Read the model definition and answer for the solid it produces. Units are mm, in the model's axes. Face numbers are marked on the shaded views. A direction names the side the tool comes from. Round coordinates to 2 decimals unless told otherwise and drop trailing zeros. Order: outer loops, then holes, each group sorted by start corner. A loop starts at its lowest first (then second) coordinate and runs counter-clockwise, first axis right, second up. Notation, with made-up numbers: (55, -5) - (112, -5) arc R22 ccw to (112, 27) - close; hole circle Ø9 at (86.5, -28). An arc over 180 degrees is marked (long way). Answer as a JSON object with one key per item and string values. Group by question number.
Q1. A cutting plane is placed at C-C on z = 29. Determine the outline of the cut face in (x, y) (3 decimals).
Q2. A cutting plane is placed at B-B on x = 45.5. Determine the outline of the cut face in (y, z), and give its area (3 significant figures).
Q3. Consider line 1 (Z direction, x = 39.5, y = -51); line 2 (Z direction, x = 9.5, y = -12); line 3 (Y direction, x = 93.5, z = 32). Determine where each line is inside the solid, lowest interval first.
Q4. Given pin 1 Ø0.9 at (x, z) = (16.5, 9.5) entering from +Y; pin 2 Ø0.6 at (x, z) = (20.5, 8.5) entering from +Y; pin 3 Ø5 at (x, z) = (18.5, 19.5) entering from +Y; pin 4 Ø4.5 at (x, z) = (108, 20.5) entering from -Y, each flat-ended and moving along its own axis, determine where each tip first touches the part or whether it passes through.
Q5. The mould has two halves that part along Z. Classify the marked faces 1, 2 and 3: pulls with the +Z half, pulls with the -Z half, needs draft (parallel to the pull), parting line crosses it, or undercut.
Q6. A tool of negligible diameter and unlimited length cuts with its end or side. For the marked faces 4 and 5, from which of +Z, -Z, +X, -X, +Y, -Y can it reach the whole face along a straight path? Write none if from no direction.
Q7. A cutting plane is placed at D-D on y = -6. Determine the outline of the cut face in (x, z) (3 decimals), and give its area (3 significant figures).
Q8. A cutting plane is placed at A-A on y = -48. Determine the outline of the cut face in (x, z) (3 decimals), and give its area (3 significant figures).
Autodesk Inventor part; units mm, degrees
ref_plane "YZ Plane" through (0, 0, 0) normal (1, 0, 0) x (0, 1, 0)
ref_plane "XZ Plane" through (0, 0, 0) normal (0, 1, 0) x (-1, 0, 0)
ref_plane "XY Plane" through (0, 0, 0) normal (0, 0, 1) x (1, 0, 0)
sketch "Sketch1" plane through (0, 0, 0) normal (0, 0, 1) x (1, 0, 0)
  line L0 (0, 0) -> (124.045, 0)
  line L1 (124.045, 0) -> (124.045, -54.7779)
  line L2 (124.045, -54.7779) -> (0, -54.7779)
  line L3 (0, -54.7779) -> (0, 0)
extrude "Extrusion1" add sketch "Sketch1" along normal blind 40
sketch "Sketch2" plane through (0, -54.7779, 0) normal (0, -1, 0) x (1, 0, 0)
  circle A0 centre (9.1512, 19.8276) radius 6.8021
  circle A1 centre (8.9796, 19.8276) radius 6.8021
  line L0 (22.4204, 25.1658) -> (80.2254, 25.1658)
  line L1 (80.2254, 25.1658) -> (80.2254, 11.439)
  line L2 (80.2254, 11.439) -> (22.4204, 11.439)
  line L3 (22.4204, 11.439) -> (22.4204, 25.1658)
  line L4 (102.3407, 25.1658) -> (111.1869, 25.1658)
  line L5 (111.1869, 25.1658) -> (111.1869, 11.439)
  line L6 (111.1869, 11.439) -> (102.3407, 11.439)
  line L7 (102.3407, 11.439) -> (102.3407, 25.1658)
  point P0 (0, 0)
  point P1 (9.0654, 26.6291)
  point P2 (9.0654, 13.026)
extrude "Extrusion2" cut sketch "Sketch2" against normal blind 40 contours A1 A0 | L0 L1 L2 L3 | L4 L5 L6 L7 picked at (6.8592, 19.8276)
sketch "Sketch3" plane through (0, 0, 0) normal (0, 1, 0) x (1, 0, 0)
  circle A0 centre (18.8298, -18.0971) radius 3.199
  arc A1 (9.0654, -26.6291) -> (9.0654, -13.026) centre (8.9796, -19.8276) ccw
  point P0 (0, 0)
extrude "Extrusion3" add sketch "Sketch3" along normal blind 4
sketch "Sketch4" plane through (18.8298, 4, 18.0971) normal (0, 1, 0) x (1, 0, 0)
  circle A0 centre (0, 0) radius 3.199
  circle A1 centre (0, 0) radius 13.6557
  point P0 (-18.8298, 18.0971)
extrude "Extrusion4" add sketch "Sketch4" along normal mid plane 2
sketch "Sketch5" plane through (18.8298, 5, 18.0971) normal (0, 1, 0) x (1, 0, 0)
  circle A0 centre (-0.2098, 8.868) radius 2.3351
  point P0 (-18.8298, 18.0971)
extrude "Extrusion5" add sketch "Sketch5" along normal blind 2
sketch "Sketch6" plane through (18.62, 7, 9.2291) normal (0, 1, 0) x (1, 0, 0)
  line L0 (1.7734, 77.6649) -> (-1.1678, 77.6649)
  line L1 (-1.1678, 77.6649) -> (-1.1678, -2.3351)
  line L2 (-1.1678, -2.3351) -> (1.7734, -2.3351)
  line L3 (1.7734, -2.3351) -> (1.7734, 77.6649)
  line L4 (1.7734, 77.6649) -> (-1.1678, -2.3351) construction
  line L5 (-1.1678, 77.6649) -> (1.7734, -2.3351) construction
  point P0 (-18.62, 9.2291)
  point P1 (0.3028, 37.6649)
  dimension "d10" = 80
extrude "Extrusion6" add sketch "Sketch6" along normal blind 2
sketch "Sketch7" plane through (0, 0, 0) normal (0, 0, -1) x (-1, 0, 0)
  point P0 (0, 0)
sketch "Sketch8" plane through (18.62, 7, 9.2291) normal (0, -1, 0) x (1, 0, 0)
  circle A0 centre (0.5375, -74.8079) radius 1.3827
  point P0 (-18.62, -9.2291)
extrude "Extrusion7" add sketch "Sketch8" along normal blind 2
properties part number "fnal"
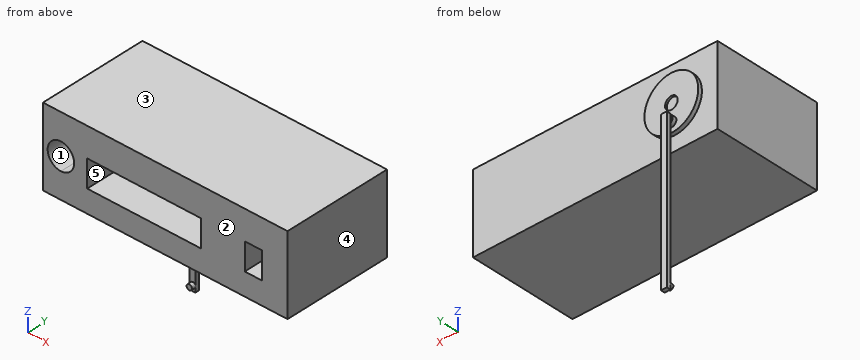
Result set:
{
 "1": {"outline": "(0, -54.778) - (124.045, -54.778) - (124.045, 0) - (0, 0) - close; (10.608, 3) - (27.052, 3) - (27.052, 5) - (10.608, 5) - close"},
 "2": {"outline": "(-54.78, 0) - (0, 0) - (0, 40) - (-54.78, 40) - (-54.78, 25.17) - (-14.78, 25.17) - (-14.78, 11.44) - (-54.78, 11.44) - close", "area": "1,640 mm²"},
 "3": {"line 1": "z = 0 to 11.44, 25.17 to 40", "line 2": "z = 0 to 40", "line 3": "y = -54.78 to 0"},
 "4": {"pin 1": "stops at y = 7", "pin 2": "stops at y = 9", "pin 3": "stops at y = 5", "pin 4": "stops at y = -14.78"},
 "5": {"face 1": "undercut", "face 2": "needs draft", "face 3": "pulls with the +Z half"},
 "6": {"face 4": "+Z, -Z, +X, +Y, -Y", "face 5": "-Y"},
 "7": {"outline": "(0, 0) - (124.045, 0) - (124.045, 40) - (0, 40) - close", "area": "4,960 mm²"},
 "8": {"outline": "(0, 0) - (124.045, 0) - (124.045, 40) - (0, 40) - close; hole (9.065, 13.026) arc R6.802 ccw to (9.065, 26.629) arc R6.802 ccw to start; hole (22.42, 11.439) - (80.225, 11.439) - (80.225, 25.166) - (22.42, 25.166) - close; hole (102.341, 11.439) - (111.187, 11.439) - (111.187, 25.166) - (102.341, 25.166) - close", "area": "3,900 mm²"}
}
